The drawing under review shows one solid part. Ordinate dimensions are in mm from its lowest x, y, z. A direction names the side the tool comes from. Give positions to 0.01 mm unless a question says otherwise; leave off trailing zeros. Write each loop counter-clockwise with the first axis right and the second up, starting at its lowest first coordinate (ties: lowest second). Pieces come first, ordered by that corner, then holes. Notation, with made-up numbers: M 86.5,82 L 126.5,82 A27 ccw 126.5,121 Z; hole C 55,64 d7. An arc over 180 degrees is marked long. Use one line per item in the form item = value. Start each with the question number.
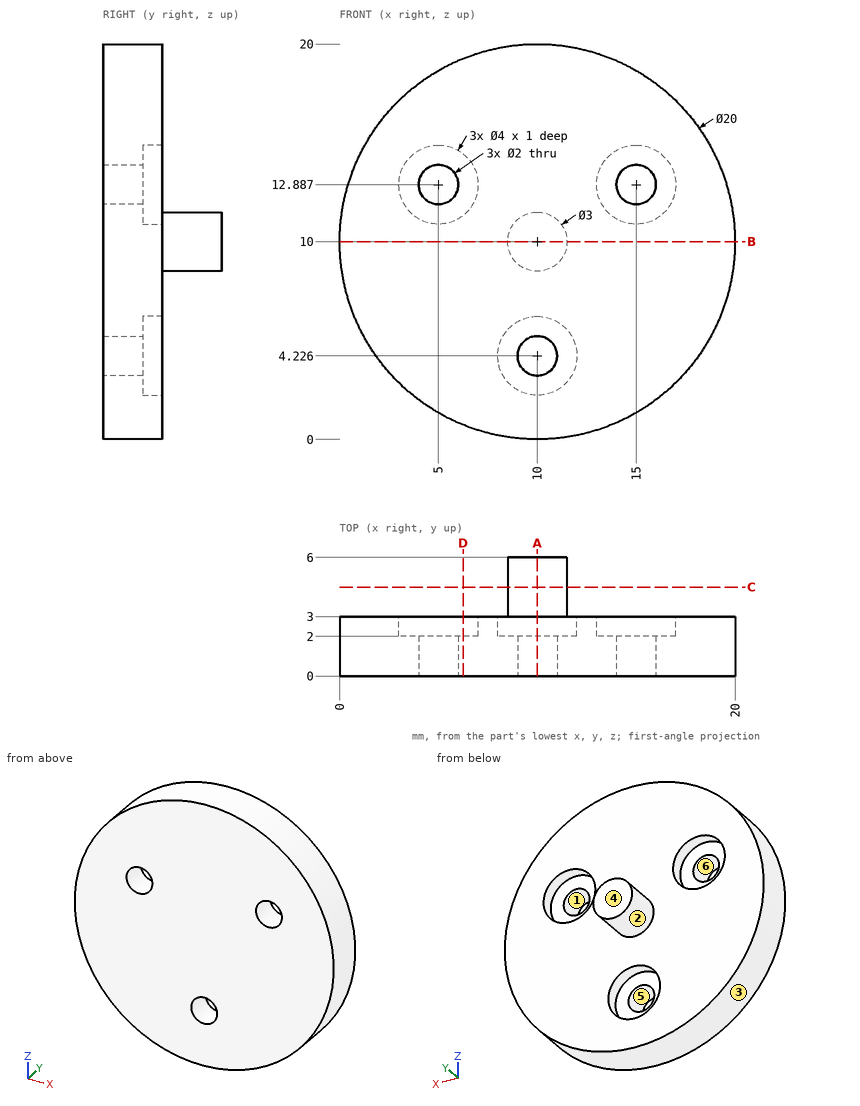
1. Clearance check with flat-ended pins moving along their axes: pin 1 Ø2.5 at (x, z) = (15, 12.89) entering from -Y; pin 2 Ø1.2 at (x, z) = (4, 12.5) entering from +Y; pin 3 Ø1.8 at (x, z) = (15, 12.89) entering from -Y; pin 4 Ø1.5 at (y, z) = (3.5, 8) entering from +X (1 decimal). State where each tip first meets the part, or that it passes through.
2. We need section B-B (z = 10). State the section outline as (x, y) points.
3. We need section D-D (x = 6.25). State the section outline as (y, z) points (1 decimal).
4. We need section C-C (y = 4.5). State the section outline as (x, z) points.
5. To check wall thickness, follow L1, parallel to Y at x = 17.5, z = 9.5; L2, parallel to Z at x = 14.25, y = 2.6; L3, parallel to X at y = 5.1, z = 10. State the ranges of each line that lie inside material, in increasing order.
6. We need section A-A (x = 10). State the section outline as (y, z) points.
7. For the marked faces 1 and 2, list the 3-axis set-ups (+Z, -Z, +X, -X, +Y, -Y) from which the entire face can be reached by the end or side of a thin tool; tool diameter is ignored.
8. Draft analysis for pull direction X (two halves, no side actions). For the marked faces 3, 4, 5 and 6, state which applies: pulls with the +X half, pulls with the -X half, needs draft (parallel to the pull), parting line crosses it, or undercut.
Answer block:
q1.pin_1 = 0
q1.pin_2 = 2
q1.pin_3 = through
q1.pin_4 = 19.9
q2.outline = M 0,0 L 20,0 L 20,3 L 11.5,3 L 11.5,6 L 8.5,6 L 8.5,3 L 0,3 Z
q3.outline = M 0,0.7 L 3,0.7 L 3,11.3 L 2,11.3 L 2,14.4 L 3,14.4 L 3,19.3 L 0,19.3 Z
q4.outline = C 10,10 d3
q5.L1 = 0 to 3
q5.L2 = 0.95 to 11.03, 14.74 to 19.05
q5.L3 = 8.5 to 11.5
q6.outline = M 0,0 L 3,0 L 3,2.23 L 2,2.23 L 2,3.23 L 0,3.23 Z; M 0,5.23 L 2,5.23 L 2,6.23 L 3,6.23 L 3,8.5 L 6,8.5 L 6,11.5 L 3,11.5 L 3,20 L 0,20 Z
q7.face_1 = +Y, -Y
q7.face_2 = +Y
q8.face_3 = parting line crosses it
q8.face_4 = needs draft
q8.face_5 = undercut
q8.face_6 = undercut
